Source: three-view drawing plus pictorial views. Frame: mm from the lowest corner of the part. A direction names the side the tool comes from. Coordinates: 2 decimals unless noted, no trailing zeros. Loops run counter-clockwise (first coordinate to the right, second up) from the corner with the lowest first, then second, coordinate; pieces in that order, holes last.
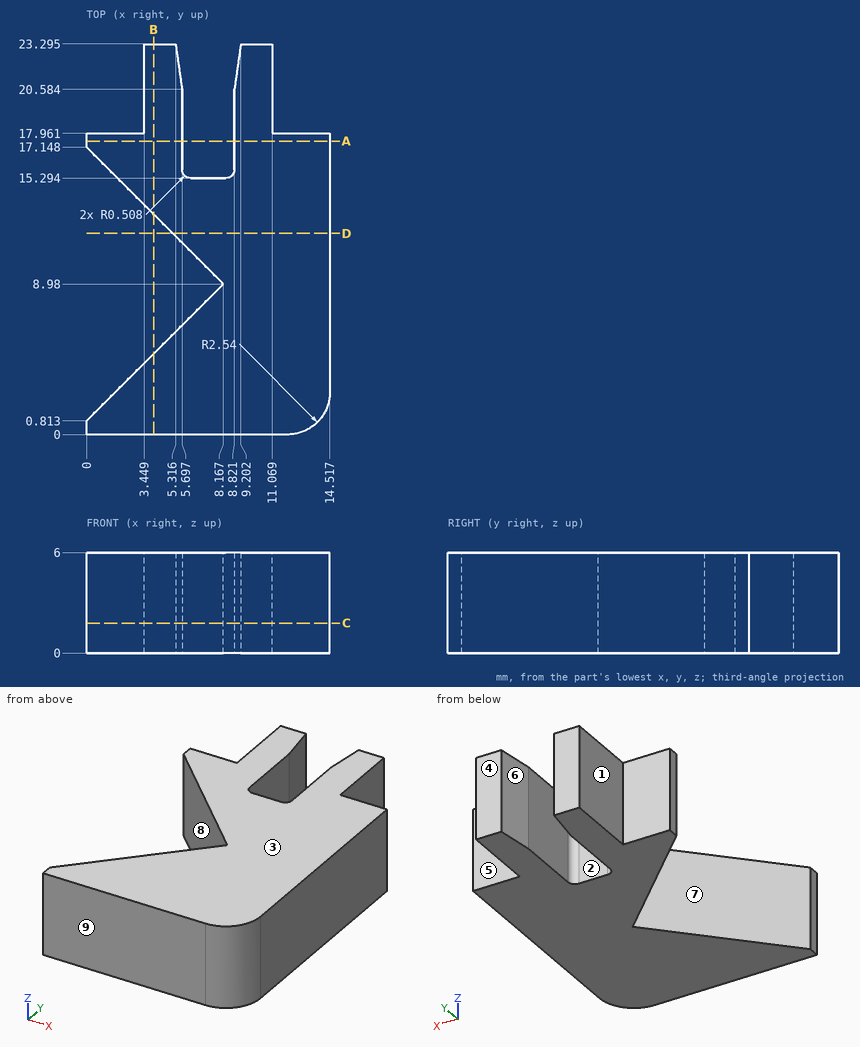
Q1. Contact query for flat-ended pins moving along their axis: pin 1 Ø2 at (x, y) = (4.5, 6.5) entering from +Z; pin 2 Ø1.6 at (y, z) = (22, 2.5) entering from -X; pin 3 Ø2.5 at (y, z) = (21, 3.5) entering from +X; pin 4 Ø1.7 at (x, z) = (1.5, 4) entering from +Y. Output: stop coordinate, or through.
Q2. Line query: line 1 along Y through (x, z) = (5.25, 4.05) (1 decimal); line 2 along X through (y, z) = (15.75, 1.85) (1 decimal); line 3 along Y through (x, z) = (3.25, 3.6) (1 decimal). Output: solid intervals per line, ascending.
Q3. Section D-D, the plane y = 12. Return the cut outline in (x, z), plus the area to 3 significant figures.
Q4. Section C-C, the plane z = 1.8. Return the cut outline in (x, y) (1 decimal).
Q5. Section A-A, the plane y = 17.5. Return the cut outline in (x, z).
Q6. Access query for the marked faces 1, 2, 3, 4 and 5. Directions: +Z, -Z, +X, -X, +Y, -Y. A direction counts if a zero-diameter tool reaches every point of the face in a straight line with its end or side. Return the directions, or none.
Q7. Section B-B, the plane x = 4. Return the cut outline in (y, z) (1 decimal).
Q8. Draft query along Y for the marked faces 6, 7, 8 and 9. Return one class per face: +Y half, -Y half, draft (parallel to the pull), parting line (faces both ways), or undercut.
Derived:
1. pin 1: stops at z = 6
1. pin 2: stops at x = 3.45
1. pin 3: stops at x = 11.07
1. pin 4: stops at y = 17.96
2. line 1: y = 0 to 6.1, 11.9 to 23.3
2. line 2: x = 1.4 to 5.7, 8.8 to 14.5
2. line 3: y = 0 to 4.1, 13.9 to 18
3. outline: (5.15, 0) - (14.52, 0) - (14.52, 6) - (5.15, 6) - close
3. area: 56.2 mm2
4. outline: (0, 0) - (12, 0) arc R2.5 ccw to (14.5, 2.5) - (14.5, 18) - (11.1, 18) - (11.1, 23.3) - (9.2, 23.3) - (8.8, 20.6) - (8.8, 15.8) arc R0.5 cw to (8.3, 15.3) - (6.2, 15.3) arc R0.5 cw to (5.7, 15.8) - (5.7, 20.6) - (5.3, 23.3) - (3.4, 23.3) - (3.4, 18) - (0, 18) - (0, 17.1) - (8.2, 9) - (0, 0.8) - close
5. outline: (0, 0) - (5.7, 0) - (5.7, 6) - (0, 6) - close; (8.82, 0) - (14.52, 0) - (14.52, 6) - (8.82, 6) - close
6. face 1: +Z, -Z, -X, +Y
6. face 2: +Z, -Z, +Y
6. face 3: +Z, +X, -X, +Y, -Y
6. face 4: +Z, -Z, +X, -X, +Y
6. face 5: +Z, -Z, +X, +Y
7. outline: (0, 0) - (4.8, 0) - (4.8, 6) - (0, 6) - close; (13.1, 0) - (23.3, 0) - (23.3, 6) - (13.1, 6) - close
8. face 6: +Y half
8. face 7: undercut
8. face 8: undercut
8. face 9: -Y half
